from build123d import *

# Parameters (mm, degrees)
F0_W     = 438
F0_H     = 612
F1_DEPTH = 915
F2_W     = 20
F2_H     = 880
F3_DEPTH = 438.001
F4_W     = 20
F4_H     = 70
F5_DEPTH = 438.001


with BuildPart() as f1:
    # F0 (on Top) → F1 (new body)
    with BuildSketch(Plane.XY):
        with Locations((-219, 306)):
            Rectangle(F0_W, F0_H)
    extrude(amount=F1_DEPTH)

    # F2 (on face) → F3 (cut, through all)
    with BuildSketch(Plane.YZ):
        with Locations((10, 440)):
            Rectangle(F2_W, F2_H)
    extrude(amount=-F3_DEPTH, mode=Mode.SUBTRACT)

    # F4 (on face) → F5 (cut, through all)
    with BuildSketch(Plane.YZ):
        with Locations((30, 35)):
            Rectangle(F4_W, F4_H)
    extrude(amount=-F5_DEPTH, mode=Mode.SUBTRACT)


solid = f1.part
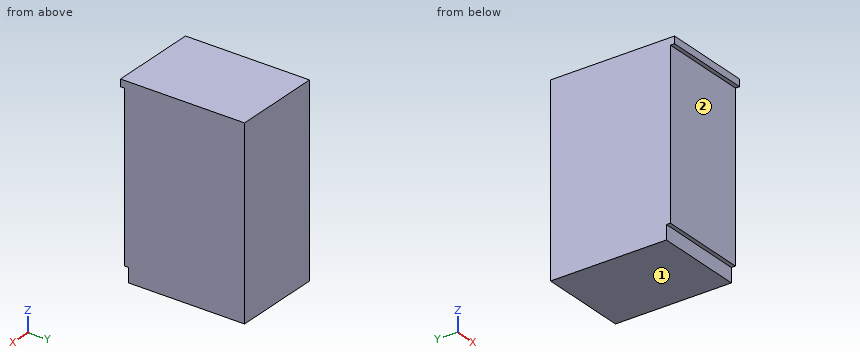
CAD build for the part. Positions are in the model's coordinates, mm. Face numbers are marked on the shaded views. A direction names the side the tool comes from. Coordinates: 2 decimals unless noted, no trailing zeros. Loops run counter-clockwise (first coordinate to the right, second up) from the corner with the lowest first, then second, coordinate; pieces in that order, holes last. Notation, with made-up numbers: (50, 66) - (96, 66) arc R27 ccw to (96, 94) - close; hole circle Ø7 at (21, 81.25). An arc over 180 degrees is marked (long way). Use one line per item in the form item = value. Start each with the question number.
1) Band-saw the part on A-A (x = -240.5). Give the cut face in (y, z).
2) Band-saw the part on B-B (z = 253). Give the cut face in (x, y).
3) Drill centre lines: L1, parallel to Y at x = -150, z = 488; L2, parallel to Z at x = -245.5, y = 34; L3, parallel to Y at x = -113, z = 44. Where is each one in solid material? Low to high. Write a range as from..to.
4) Flat gauge pins, fed straight in: pin 1 (16 mm diameter, centred on x = -244.5, y = 28.5, fed in from -Z); pin 2 (6 mm diameter, centred on x = -190, y = 12, fed in from -Z); pin 3 (5 mm diameter, centred on x = -108.5, z = 264, fed in from -Y). Where does each tip first touch, or does it go through?
5) Tool access for the marked faces 1 and 2: list every direction of +Z, -Z, +X, -X, +Y, -Y with a clear straight run to the whole face (end or side of a thin tool).
Check values:
q1.outline = (0, 880) - (20, 880) - (20, 70) - (40, 70) - (40, 0) - (612, 0) - (612, 915) - (0, 915) - close
q2.outline = (-438, 20) - (0, 20) - (0, 612) - (-438, 612) - close
q3.L1 = 20..612
q3.L2 = 70..915
q3.L3 = 40..612
q4.pin_1 = 70
q4.pin_2 = 880
q4.pin_3 = 20
q5.face_1 = -Z, +X, -X, +Y, -Y
q5.face_2 = -Z, +X, -X, -Y
